Part model, mm, in its own coordinate system. A direction names the side the tool comes from. Coordinates: 2 decimals unless noted, no trailing zeros. Write each loop counter-clockwise with the first axis right and the second up, starting at its lowest first coordinate (ties: lowest second). Pieces come first, ordered by that corner, then holes. Notation, with made-up numbers: M 32.5,30.5 L 45.5,30.5 A24 cw 45.5,45.5 Z; hole C 18,-21.75 d2. An arc over 180 degrees is marked long. Use a Markdown table: item, result. Add a question column.
Q1. Slice it at C-C on x = -13. Write the cut outline in (y, z).
Q2. Slice it at A-A on y = 90.25. Write the cut outline in (x, z).
Q3. Wall check: L1, parallel to X at y = 89.5, z = 98.25; L2, parallel to Y at x = -14.5, z = 110.5; L3, parallel to X at y = 90, z = 106. Give the ranges that are in metal, low to high. Write a range as from..to.
Q4. Slice it at D-D on z = 107. Write the cut outline in (x, y), then the cut area to 3 significant figures.
Q5. Mould opens along X. For faces 1 (the flat face through (-8.251, 90, 101)), 2 (the flat face through (-9.051, 90, 98)), 3 (the flat face through (-12, 90, 114.335)) say: released by +X, released by -X, zero draft, split by the parting line, or undercut.
Q6. Tool access for faces 4 (the flat face through (-12, 86.916, 98)), 5 (the flat face through (-9.451, 90, 109)), 6 (the flat face through (-12.19, 92.21, 113.84)), 7 (the flat face through (-12, 87.316, 109)), 8 (the flat face through (-14.344, 89.978, 113.842)): list every direction of +Z, -Z, +X, -X, +Y, -Y with a clear straight run to the whole face (end or side of a thin tool).
Q7. Pin check, flat tips, straight feed: pin 1 Ø3 at (y, z) = (92, 108) entering from +X; pin 2 Ø4.5 at (y, z) = (90.5, 111) entering from -X; pin 3 Ø1 at (x, y) = (-11, 90) entering from -Z. Stop position of each tip, or through.
Q8. Slice it at B-B on z = 100. Write the cut outline in (x, y).
from build123d import *

# Parameters (mm, degrees)
SKETCH2_W           = 7.799999809
SKETCH2_H           = 7.79999981
BOSS_EXTRUDE1_DEPTH = 5
SKETCH3_W           = 7.799999809
SKETCH3_H           = 7.79999981
SKETCH3_W_2         = 6.199999809
SKETCH3_H_2         = 6.19999981
BOSS_EXTRUDE2_DEPTH = 4
SKETCH4_W           = 5.399999809
SKETCH4_H           = 5.39999981
BOSS_EXTRUDE3_DEPTH = 9
CHAMFER1_SIZE       = 1


with BuildPart() as part:
    # Sketch2 → Boss-Extrude1 (new body)
    with BuildSketch(Plane.XY.offset(100.335422766)):
        with Locations((-12.150804877, 90.015849294)):
            Rectangle(SKETCH2_W, SKETCH2_H)
    extrude(amount=BOSS_EXTRUDE1_DEPTH)

    # Sketch3 → Boss-Extrude2 (add)
    with BuildSketch(Plane(origin=(0, 0, 100.335422766), x_dir=(-1, 0, 0), z_dir=(0, 0, -1))):
        with Locations((12.150804877, 90.015849294)):
            Rectangle(SKETCH3_W, SKETCH3_H)
        with Locations((12.150804877, 90.015849294)):
            Rectangle(SKETCH3_W_2, SKETCH3_H_2, mode=Mode.SUBTRACT)
    extrude(amount=BOSS_EXTRUDE2_DEPTH)

    # Sketch4 → Boss-Extrude3 (add)
    with BuildSketch(Plane.XY.offset(105.335422766)):
        with Locations((-12.150804877, 90.015849294)):
            Rectangle(SKETCH4_W, SKETCH4_H)
    extrude(amount=BOSS_EXTRUDE3_DEPTH)

    # Chamfer1
    chamfer1_edges = [part.edges().sort_by_distance(p)[0] for p in [
        (-14.850804781, 90.015849294, 114.335422766),
        (-12.150804876, 87.315849389, 114.335422766),
        (-9.450804972, 90.015849294, 114.335422766),
        (-12.150804876, 92.715849199, 114.335422766),
    ]]
    chamfer(chamfer1_edges, length=CHAMFER1_SIZE)


solid = part.part
Recorded:
| question | item | result |
|---|---|---|
| 1 | outline | M 86.12,96.34 L 86.92,96.34 L 86.92,100.34 L 93.12,100.34 L 93.12,96.34 L 93.92,96.34 L 93.92,105.34 L 92.72,105.34 L 92.72,113.34 L 91.72,114.34 L 88.32,114.34 L 87.32,113.34 L 87.32,105.34 L 86.12,105.34 Z |
| 2 | outline | M -16.05,96.34 L -15.25,96.34 L -15.25,100.34 L -9.05,100.34 L -9.05,96.34 L -8.25,96.34 L -8.25,105.34 L -9.45,105.34 L -9.45,113.34 L -10.45,114.34 L -13.85,114.34 L -14.85,113.34 L -14.85,105.34 L -16.05,105.34 Z |
| 3 | L1 | -16.05..-15.25, -9.05..-8.25 |
| 3 | L2 | 87.32..92.72 |
| 3 | L3 | -14.85..-9.45 |
| 4 | outline | M -14.85,87.32 L -9.45,87.32 L -9.45,92.72 L -14.85,92.72 Z |
| 4 | area | 29.2 mm² |
| 5 | face 1 | released by +X |
| 5 | face 2 | undercut |
| 5 | face 3 | zero draft |
| 6 | face 4 | -Z |
| 6 | face 5 | +Z, +X, +Y, -Y |
| 6 | face 6 | +Z, +X, -X, +Y |
| 6 | face 7 | +Z, +X, -X, -Y |
| 6 | face 8 | +Z, -X, +Y, -Y |
| 7 | pin 1 | x = -9.45 |
| 7 | pin 2 | x = -14.85 |
| 7 | pin 3 | z = 100.34 |
| 8 | outline | M -16.05,86.12 L -8.25,86.12 L -8.25,93.92 L -16.05,93.92 Z; hole M -15.25,86.92 L -9.05,86.92 L -9.05,93.12 L -15.25,93.12 Z |
